Autodesk Inventor part; units mm, degrees
ref_plane "YZ Plane" through (0, 0, 0) normal (1, 0, 0) x (0, 1, 0)
ref_plane "XZ Plane" through (0, 0, 0) normal (0, 1, 0) x (-1, 0, 0)
ref_plane "XY Plane" through (0, 0, 0) normal (0, 0, 1) x (1, 0, 0)
sketch "Sketch1" plane through (0, 0, 0) normal (1, 0, 0) x (0, 1, 0)
  line L0 (0, 0) -> (50.8, 0)
  line L1 (50.8, 0) -> (50.8, -50.8)
  line L2 (50.8, -50.8) -> (0, -50.8)
  line L3 (0, -50.8) -> (0, 0)
  line L4 (50.8, 0) -> (50.8, -25.4)
  circle A0 centre (25.4, -25.4) radius 4.0132
  dimension "d0" = 50.8
  dimension "d1" = 50.8
  dimension "d5" = 8.0264
extrude "Extrusion1" add sketch "Sketch1" along normal blind 11.43
sketch "Sketch2" plane through (11.43, 0, 0) normal (1, 0, 0) x (0, 0, -1)
  line L0 (12.319, 38.481) -> (38.481, 38.481)
  line L1 (38.481, 38.481) -> (38.481, 12.319)
  line L2 (38.481, 12.319) -> (12.319, 12.319)
  line L3 (12.319, 12.319) -> (12.319, 38.481)
  line L4 (50.8, 50.8) -> (0, 50.8)
  line L5 (0, 0) -> (50.8, 0)
  line L6 (0, 50.8) -> (0, 0)
  dimension "d8" = 26.162
  dimension "d9" = 26.162
extrude "Extrusion2" cut sketch "Sketch2" against normal blind 3.048
sketch "Sketch3" plane through (0, 0, 0) normal (-1, 0, 0) x (0, 0, 1)
  circle A0 centre (-25.4, 25.4) radius 4.0132
  circle A1 centre (-25.4, 25.4) radius 8.255
  point P0 (0, 0)
  dimension "d12" = 16.51
extrude "Extrusion3" cut sketch "Sketch3" against normal blind 1.905
sketch "Sketch4" plane through (0, 0, 0) normal (0, 0, 1) x (1, 0, 0)
  line L0 (0, 0) -> (11.43, 0)
  line L1 (0, 50.8) -> (11.43, 50.8)
  line L2 (0, 0) -> (5.08, 0)
  line L3 (5.08, 0) -> (5.08, 50.8)
  line L4 (5.08, 50.8) -> (0, 50.8)
  line L5 (0, 50.8) -> (0, 0)
  dimension "d15" = 5.08
extrude "Extrusion4" cut sketch "Sketch4" against normal blind 50.8
properties part number "220425 End Cap"
The listing builds one solid part. Answer for the finished solid, in the listing's coordinates (mm). A direction names the side the tool comes from. Give positions to 0.01 mm unless a question says otherwise; leave off trailing zeros. Loops run counter-clockwise (first coordinate to the right, second up) from the corner with the lowest first, then second, coordinate; pieces in that order, holes last. Notation, with made-up numbers: M -25.5,32 L 27.5,32 A6 cw 27.5,37 Z; hole C -4,48 d4. An arc over 180 degrees is marked long. One line per item, written item: value.
Q1. A cutting plane is placed at C-C on x = 9. Determine the outline of the cut face in (y, z), then the cut area to 3 significant figures.
Working result:
outline: M 0,-50.8 L 50.8,-50.8 L 50.8,0 L 0,0 Z; hole M 12.32,-38.48 L 38.48,-38.48 L 38.48,-12.32 L 12.32,-12.32 Z
area: 1,900 mm^2
Q2. For faces 1 (the face through (10, 38.481, -25)), 2 (the face through (6.71, 21.39, -25.58)), determine the directions among +Z, -Z, +X, -X, +Y, -Y from which every point of the face is accessible in a straight line to the end or side of a thin tool.
Working result:
face 1: +X
face 2: +X, -X
Q3. Find the intervals of material crossed by line 1 (Z direction, x = 9.25, y = 23); line 2 (Y direction, x = 9.75, z = -33); line 3 (Y direction, x = 6.95, z = -25.4), in increasing order. Write a range as from..to.
Working result:
line 1: z = -50.8..-38.48, -12.32..0
line 2: y = 0..12.32, 38.48..50.8
line 3: y = 0..21.39, 29.41..50.8
Q4. Determine the mould class of faces 3 (the face through (10, 12.319, -26)), 4 (the face through (8, 50.8, -25)), 5 (the face through (10, 26, -38.481)), 6 (the face through (8, 25, 0)) for opening direction Y: +Y half, -Y half, draft (parallel to the pull), parting line (faces both ways), or undercut.
Working result:
face 3: undercut
face 4: +Y half
face 5: undercut
face 6: draft
Q5. A flat-ended cylindrical pin translates along its axis: P1, Ø8, axis at y = 30, z = -30.5, coming from the +X side. Find the tip coordinate at first contact, or state that the pin passes through.
Working result:
P1: stops at x = 8.38
Q6. A cutting plane is placed at D-D on z = -31. Determine the outline of the cut face in (x, y).
Working result:
outline: M 5.08,0 L 11.43,0 L 11.43,12.32 L 8.38,12.32 L 8.38,38.48 L 11.43,38.48 L 11.43,50.8 L 5.08,50.8 Z
Q7. A cutting plane is placed at B-B on y = 25.4. Determine the outline of the cut face in (x, z), then the cut area to 3 significant figures.
Working result:
outline: M 5.08,-50.8 L 11.43,-50.8 L 11.43,-38.48 L 8.38,-38.48 L 8.38,-29.41 L 5.08,-29.41 Z; M 5.08,-21.39 L 8.38,-21.39 L 8.38,-12.32 L 11.43,-12.32 L 11.43,0 L 5.08,0 Z
area: 216 mm^2
Q8. A cutting plane is placed at A-A on z = -25.4. Determine the outline of the cut face in (x, y).
Working result:
outline: M 5.08,0 L 11.43,0 L 11.43,12.32 L 8.38,12.32 L 8.38,21.39 L 5.08,21.39 Z; M 5.08,29.41 L 8.38,29.41 L 8.38,38.48 L 11.43,38.48 L 11.43,50.8 L 5.08,50.8 Z
